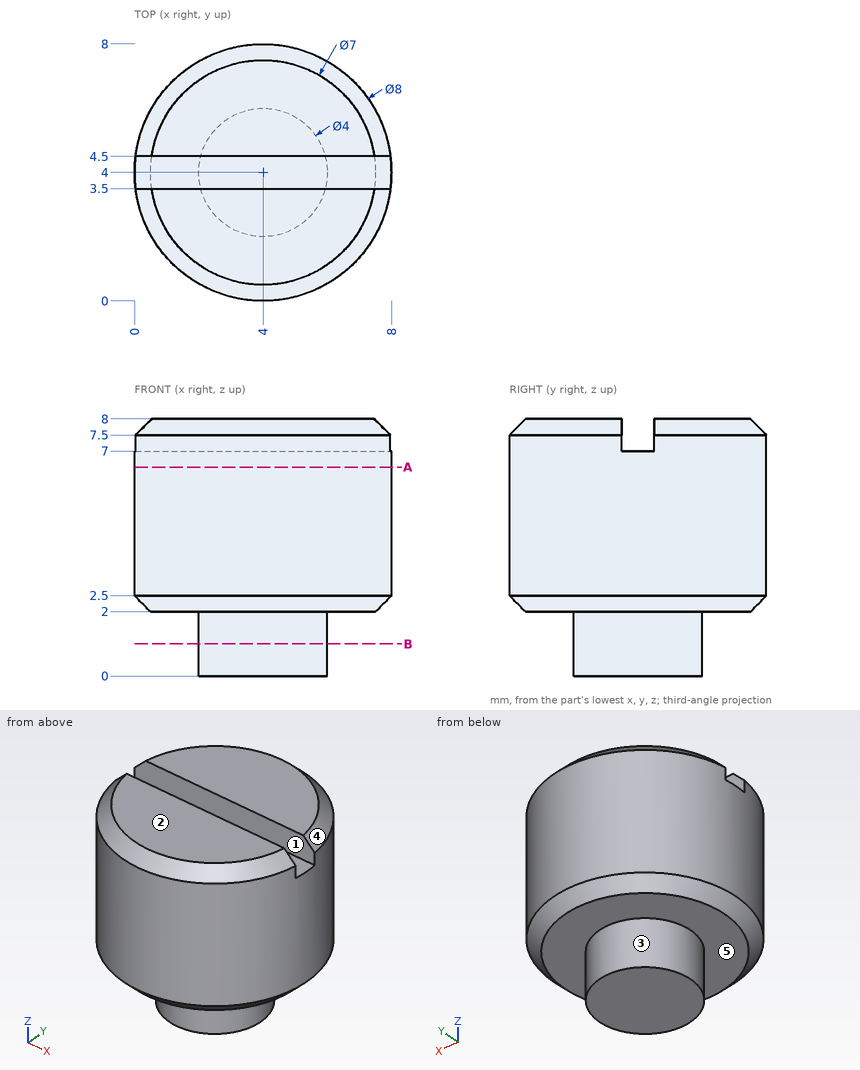
The drawing under review shows one solid part. Ordinate dimensions are in mm from its lowest x, y, z. A direction names the side the tool comes from. Coordinates: 2 decimals unless noted, no trailing zeros. Loops run counter-clockwise (first coordinate to the right, second up) from the corner with the lowest first, then second, coordinate; pieces in that order, holes last. Notation, with made-up numbers: M 47,69.25 L 53,69.25 A13 ccw 53,74.25 Z; hole C 61.5,65.5 d10. An arc over 180 degrees is marked long. Use one line per item in the form item = value.
(1) For the marked faces 4 and 5, list the 3-axis set-ups (+Z, -Z, +X, -X, +Y, -Y) from which the entire face can be reached by the end or side of a thin tool; tool diameter is ignored.
Return value:
face_4 = +Z, +Y
face_5 = -Z
(2) Consider section A-A (z = 6.5). Write out the cut boundary in (x, y), and give its area (3 significant figures).
Return value:
outline = C 4,4 d8
area = 50.3 mm2
(3) Clearance check with flat-ended pins moving along their axes: P1, Ø0.5, axis at x = 4.5, z = 7.5, coming from the -Y side; P2, Ø3, axis at y = 1, z = 1.5, coming from the +X side. State where each tip first meets the part, or that it passes through.
Return value:
P1 = 0.01
P2 = 7.53
(4) Consider section B-B (z = 1). Write out the cut boundary in (x, y), and give its area (3 significant figures).
Return value:
outline = C 4,4 d4
area = 12.6 mm2
(5) Draft analysis for pull direction Y (two halves, no side actions). For the marked faces 1, 2 and 3, state which applies: pulls with the +Y half, pulls with the -Y half, needs draft (parallel to the pull), parting line crosses it, or undercut.
Return value:
face_1 = undercut
face_2 = needs draft
face_3 = parting line crosses it
(6) For line 1 along X through (y, z) = (3.5, 5); line 2 along Z through (x, y) = (3.75, 1.25); line 3 along Z through (x, y) = (3, 4.25), list the stretches that pass through material, from the lowest coordinate up. Write a range as from..to.
Return value:
line_1 = 0.03..7.97
line_2 = 2..8
line_3 = 0..7
